Geometry check sheet. Reference: drawing and pictorial views, mm from the part's lowest x, y, z. Coordinates: 2 decimals unless noted, no trailing zeros. Put each result on its own line as item: value.
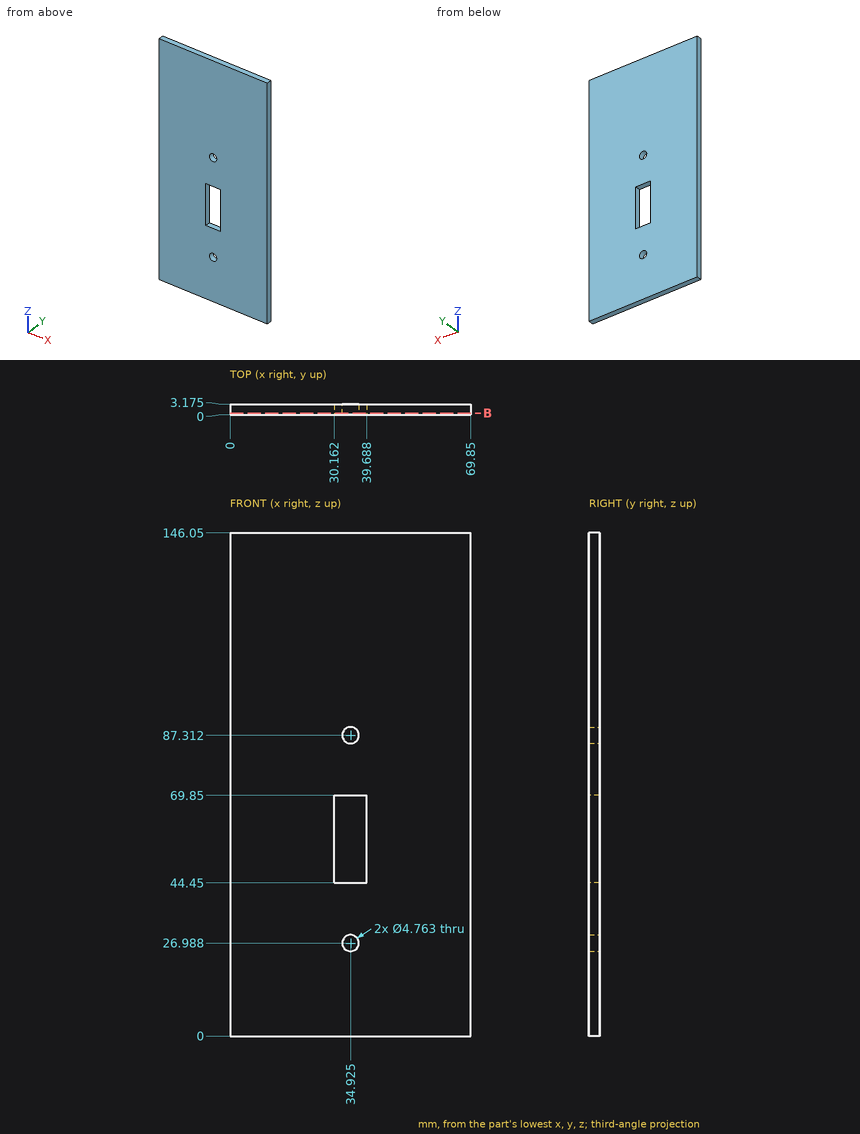
Q1. Depth check by flat-ended pin: P1, Ø4, axis at x = 34.92, z = 87.31, coming from the +Y side. Enter the tip coordinate at first touch or a pass-through.
Recorded:
P1: passes through
Q2. Material ranges on line 1 along X through (y, z) = (2.85, 69.5); line 2 along Z through (x, y) = (39, 1.15), recorded low to high.
Recorded:
line 1: x = 0 to 30.16, 39.69 to 69.85
line 2: z = 0 to 44.45, 69.85 to 146.05
Q3. Cross-section at B-B (y = 0.5). State how many separate pieces and enclosed holes the cut face has, plus the area to 3 significant figures.
Recorded:
separate pieces: 1
enclosed holes: 3
area: 9,920 mm2
